CAD build for the part. Positions are in the model's coordinates, mm. A direction names the side the tool comes from. Give positions to 0.01 mm unless a question says otherwise; leave off trailing zeros. Write item = value, one per line. Start each with the question number.
```python
from build123d import *

# Parameters (mm, degrees)
BOSS_EXTRUDE1_DEPTH = 1.5
CUT_EXTRUDE1_DEPTH  = 2
SKETCH3_R           = 4
CUT_EXTRUDE2_DEPTH  = 2
SKETCH4_R           = 20
CUT_EXTRUDE3_DEPTH  = 0.5
FILLET1_R           = 1
SKETCH5_R           = 22
BOSS_EXTRUDE2_DEPTH = 3
SKETCH6_R           = 6.5
BOSS_EXTRUDE3_DEPTH = 2
CHAMFER1_SIZE       = 0.5
CHAMFER1_SIZE2      = 0.288675135
SKETCH7_R           = 7.5
BOSS_EXTRUDE4_DEPTH = 1.5
SKETCH8_R           = 22
BOSS_EXTRUDE5_DEPTH = 7
FILLET3_R           = 2
CUT_EXTRUDE4_START  = -3
SKETCH9_R           = 8
SKETCH9_R_2         = 6.5
CUT_EXTRUDE4_DEPTH  = 3
FILLET4_R           = 3


# Some blends are built 0.0001 mm under size
with BuildPart() as part:
    # Sketch1 → Boss-Extrude1 (new body)
    with BuildSketch(Plane(origin=(0, 0, 0), x_dir=(1, 0, 0), z_dir=(0, 1, 0))):
        with BuildLine():
            Line((-20.5, -35), (20.5, -35))
            ThreePointArc((20.5, -35), (24.035533906, -33.535533906), (25.5, -30))
            Line((25.5, -30), (25.5, 30))
            ThreePointArc((25.5, 30), (24.035533906, 33.535533906), (20.5, 35))
            Line((20.5, 35), (-20.5, 35))
            ThreePointArc((-20.5, 35), (-24.035533906, 33.535533906), (-25.5, 30))
            Line((-25.5, 30), (-25.5, -30))
            ThreePointArc((-25.5, -30), (-24.035533906, -33.535533906), (-20.5, -35))
        make_face()
    extrude(amount=BOSS_EXTRUDE1_DEPTH)

    # Sketch2 → Cut-Extrude1 (cut)
    with BuildSketch(Plane(origin=(0, 1.5, 0), x_dir=(1, 0, 0), z_dir=(0, 1, 0))):
        with BuildLine():
            Line((-21.5, 24.5), (-21.5, 28.5))
            ThreePointArc((-21.5, 28.5), (-17.5, 32.5), (-13.5, 28.5))
            Line((-13.5, 28.5), (-13.5, 24.5))
            ThreePointArc((-13.5, 24.5), (-17.5, 20.5), (-21.5, 24.5))
        make_face()
        with BuildLine():
            Line((13.5, 24.5), (13.5, 28.5))
            ThreePointArc((13.5, 28.5), (17.5, 32.5), (21.5, 28.5))
            Line((21.5, 28.5), (21.5, 24.5))
            ThreePointArc((21.5, 24.5), (17.5, 20.5), (13.5, 24.5))
        make_face()
    cut_extrude1 = extrude(amount=-CUT_EXTRUDE1_DEPTH, mode=Mode.SUBTRACT)

    # Mirror1: Cut-Extrude1 across plane
    add(cut_extrude1.mirror(Plane.XY), mode=Mode.SUBTRACT)

    # Sketch3 → Cut-Extrude2 (cut)
    with BuildSketch(Plane(origin=(0, 1.5, 0), x_dir=(1, 0, 0), z_dir=(0, 1, 0))):
        with Locations(Location((0, 0, 0), (0, 0, 270))):
            Circle(SKETCH3_R)
    extrude(amount=-CUT_EXTRUDE2_DEPTH, mode=Mode.SUBTRACT)

    # Sketch4 → Cut-Extrude3 (cut)
    with BuildSketch(Plane(origin=(0, 1.5, 0), x_dir=(1, 0, 0), z_dir=(0, 1, 0))):
        with Locations(Location((0, 0, 0), (0, 0, 270))):
            Circle(SKETCH4_R)
    extrude(amount=-CUT_EXTRUDE3_DEPTH, mode=Mode.SUBTRACT)

    # Fillet1
    # the kernel refuses this fillet: 1 mm, written as the material it takes off along each edge
    with BuildSketch(Plane(origin=(0, 1.5, 0), x_dir=(0, 0, 1), z_dir=(-1, 0, 0))) as fillet1_piece_1:
        with BuildLine():
            CenterArc((20.866025404, -1), FILLET1_R, 90, 60)
            Line((20, -0.5), (19.982679492, -0.49))
            ThreePointArc((19.982679492, -0.49), (19.98, -0.25), (19.98, 0))
            Line((19.98, 0), (20, 0.02))
            Line((20, 0.02), (20.866025404, 0.02))
            Line((20.866025404, 0.02), (20.866025404, 0))
        make_face()
    revolve(axis=Axis((0, 1.5, 0), (0, 1, 0)), mode=Mode.SUBTRACT)

    # Sketch5 → Boss-Extrude2 (add)
    with BuildSketch(Plane.XZ):
        with Locations(Location((0, 0, 0), (0, 0, 270))):
            Circle(SKETCH5_R)
    extrude(amount=BOSS_EXTRUDE2_DEPTH)

    # Sketch6 → Boss-Extrude3 (add)
    with BuildSketch(Plane(origin=(0, 1, 0), x_dir=(1, 0, 0), z_dir=(0, 1, 0))):
        with Locations(Location((0, 0, 0), (0, 0, 270))):
            Circle(SKETCH6_R)
    extrude(amount=BOSS_EXTRUDE3_DEPTH)

    # Chamfer1
    chamfer1_edges = [part.edges().sort_by_distance(p)[0] for p in [
        (0, 3, -6.5),
    ]]
    chamfer1_side = [part.faces().sort_by_distance(p)[0] for p in [
        (0, 2, -6.5),
    ]]
    chamfer(chamfer1_edges, length=CHAMFER1_SIZE, length2=CHAMFER1_SIZE2, reference=chamfer1_side[0])

    # Sketch7 → Boss-Extrude4 (add)
    with BuildSketch(Plane.XZ.offset(3)):
        with Locations(Location((0, 0, 0), (0, 0, 270))):
            Circle(SKETCH7_R)
    extrude(amount=BOSS_EXTRUDE4_DEPTH)

    # Sketch8 → Boss-Extrude5 (add)
    with BuildSketch(Plane.XZ.offset(4.5)):
        with Locations(Location((0, 0, 0), (0, 0, 270))):
            Circle(SKETCH8_R)
    extrude(amount=BOSS_EXTRUDE5_DEPTH)

    # Fillet3
    fillet3_edges = [part.edges().sort_by_distance(p)[0] for p in [
        (0, -11.5, 22),
    ]]
    fillet(fillet3_edges, radius=FILLET3_R)

    # Sketch9 → Cut-Extrude4 (cut)
    with BuildSketch(Plane(origin=(0, 1, 0), x_dir=(1, 0, 0), z_dir=(0, 1, 0)).offset(CUT_EXTRUDE4_START)):
        with Locations(Location((0, 0, 0), (0, 0, 270))):
            Circle(SKETCH9_R)
        with Locations(Location((0, 0, 0), (0, 0, 270))):
            Circle(SKETCH9_R_2, mode=Mode.SUBTRACT)
    extrude(amount=CUT_EXTRUDE4_DEPTH, mode=Mode.SUBTRACT)

    # Fillet4
    fillet4_edges = [part.edges().sort_by_distance(p)[0] for p in [
        (0, 1, -8),
    ]]
    fillet(fillet4_edges, radius=FILLET4_R - 0.0001)  # a hair under: the kernel refuses the full size


solid = part.part
```
1. Pin check, flat tips, straight feed: pin 1 Ø4 at (x, z) = (-15.5, 16) entering from +Y; pin 2 Ø1.5 at (y, z) = (-9.5, -20) entering from +X; pin 3 Ø1.5 at (y, z) = (-2, 25.5) entering from +X; pin 4 Ø2 at (x, z) = (-5.5, 5) entering from +Y. Stop position of each tip, or through.
2. Wall check: line 1 along X through (y, z) = (-1.95, 0); line 2 along Z through (x, y) = (1.5, 1.25); line 3 along Y through (x, z) = (-16, 9). Give the ranges that are in metal, low to high.
3. Tool access for faces 1 (the flat face through (7, -2, 0)), 2 (the cylindrical face through (17.6, 0.8, 20.5)), 3 (the cylindrical face through (-21.477, -6.965, 4.769)): list every direction of +Z, -Z, +X, -X, +Y, -Y with a clear straight run to the whole face (end or side of a thin tool).
4. Cut at A-A (x = 17.5). Count the separate pieces of the cut face and the enclosed holes in it, then the cut area to 3 significant figures.
5. Mould opens along Y. For faces 4 (the cylindrical face through (-17.4, 0.8, 20.5)), 5 (the flat face through (22.3, 0, -0.5)), 6 (the cylindrical face through (-3.905, 0.507, -0.867)) say: +Y half, -Y half, draft (parallel to the pull), parting line (faces both ways), or undercut.
Output:
q1.pin_1 = 1.5
q1.pin_2 = 10.65
q1.pin_3 = through
q1.pin_4 = 2.62
q2.line_1 = -22 to -8, -6.5 to 6.5, 8 to 22
q2.line_2 = -35 to -20.15, -6.32 to 6.32, 20.15 to 35
q2.line_3 = -11.5 to -4.5, -3 to 1
q3.face_1 = +Y
q3.face_2 = +Y, -Y
q3.face_3 = -Y
q4.separate_pieces = 4
q4.enclosed_holes = 0
q4.area = 323 mm2
q5.face_4 = draft
q5.face_5 = -Y half
q5.face_6 = undercut
